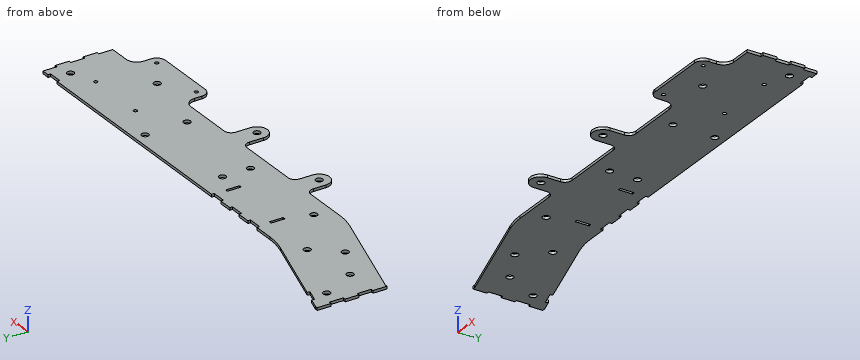
from build123d import *

# Parameters (mm, degrees)
SKETCH2_R                           = 6.35
BASE_DEPTH                          = 4.826
SKETCH3_W                           = 4.826
SKETCH3_H                           = 25.4
CENTER_SUPPORT_VERTICAL_HOLES_DEPTH = 5.826
SKETCH4_W                           = 4.826
SKETCH4_H                           = 25.4
CUT_EXTRUDE2_DEPTH                  = 9.652
SKETCH5_R                           = 3.3528
BOSS_EXTRUDE1_DEPTH                 = 4.826
SKETCH6_R                           = 3.3528
CUT_EXTRUDE3_DEPTH                  = 5.826
SKETCH7_W                           = 25.4
SKETCH7_H                           = 4.826
CUT_EXTRUDE4_DEPTH                  = 4.826


with BuildPart() as part:
    # Sketch2 → base (new body)
    with BuildSketch(Plane.XY):
        with BuildLine():
            Line((-214.699698696, -160.199792202), (-26.873942154, -218.069670807))
            ThreePointArc((-26.873942154, -218.069670807), (-8.387395977, -222.284374422), (10.520610491, -223.699792202))
            Line((10.520610491, -223.699792202), (91.809301303, -223.699792202))
            ThreePointArc((91.809301303, -223.699792202), (100.789557424, -227.419536081), (104.509301303, -236.399792202))
            Line((104.509301303, -236.399792202), (104.509301303, -259.444792203))
            ThreePointArc((104.509301303, -259.444792203), (123.559301303, -278.494792203), (142.609301303, -259.444792203))
            Line((142.609301303, -259.444792203), (142.609301303, -236.399792202))
            ThreePointArc((142.609301303, -236.399792202), (146.329045182, -227.419536081), (155.309301303, -223.699792202))
            Line((155.309301303, -223.699792202), (271.099301303, -223.699792202))
            ThreePointArc((271.099301303, -223.699792202), (280.079557424, -227.419536081), (283.799301303, -236.399792202))
            Line((283.799301303, -236.399792202), (283.799301303, -262.624792203))
            ThreePointArc((283.799301303, -262.624792203), (302.849301303, -281.674792203), (321.899301303, -262.624792203))
            Line((321.899301303, -262.624792203), (321.899301303, -236.399792202))
            ThreePointArc((321.899301303, -236.399792202), (325.619045182, -227.419536081), (334.599301303, -223.699792202))
            Line((334.599301303, -223.699792202), (476.201681216, -223.699792202))
            ThreePointArc((476.201681216, -223.699792202), (482.250146931, -225.232605336), (486.838586238, -229.461042202))
            ThreePointArc((486.838586238, -229.461042202), (518.749301303, -246.744792203), (550.660016368, -229.461042202))
            ThreePointArc((550.660016368, -229.461042202), (555.248455675, -225.232605336), (561.29692139, -223.699792202))
            Line((561.29692139, -223.699792202), (656.774301304, -223.699792202))
            Line((656.774301304, -223.699792202), (656.774301304, -198.299792202))
            Line((656.774301304, -198.299792202), (651.948301304, -198.299792202))
            Line((651.948301304, -198.299792202), (651.948301304, -172.899792202))
            Line((651.948301304, -172.899792202), (656.774301304, -172.899792202))
            Line((656.774301304, -172.899792202), (656.774301304, -147.499792202))
            Line((656.774301304, -147.499792202), (651.948301304, -147.499792202))
            Line((651.948301304, -147.499792202), (651.948301304, -122.099792202))
            Line((651.948301304, -122.099792202), (656.774301304, -122.099792202))
            Line((656.774301304, -122.099792202), (656.774301304, -96.699792202))
            Line((656.774301304, -96.699792202), (174.174301304, -96.699792202))
            Line((174.174301304, -96.699792202), (174.174301304, -101.525792202))
            Line((174.174301304, -101.525792202), (148.774301304, -101.525792202))
            Line((148.774301304, -101.525792202), (148.774301304, -96.699792202))
            Line((148.774301304, -96.699792202), (123.374301304, -96.699792202))
            Line((123.374301304, -96.699792202), (123.374301304, -101.525792202))
            Line((123.374301304, -101.525792202), (97.974301304, -101.525792202))
            Line((97.974301304, -101.525792202), (97.974301304, -96.699792202))
            Line((97.974301304, -96.699792202), (72.574301304, -96.699792202))
            Line((72.574301304, -96.699792202), (72.574301304, -101.525792202))
            Line((72.574301304, -101.525792202), (47.174301304, -101.525792202))
            Line((47.174301304, -101.525792202), (47.174301304, -96.699792202))
            Line((47.174301304, -96.699792202), (10.520610491, -96.699792202))
            ThreePointArc((10.520610491, -96.699792202), (-8.387395977, -95.284374422), (-26.873942154, -91.069670807))
            Line((-26.873942154, -91.069670807), (-169.556754254, -47.108516771))
            Line((-169.556754254, -47.108516771), (-170.977747254, -51.720572158))
            Line((-170.977747254, -51.720572158), (-195.251722975, -44.241661629))
            Line((-195.251722975, -44.241661629), (-193.830729974, -39.629606242))
            Line((-193.830729974, -39.629606242), (-214.699698696, -33.199792202))
            Line((-214.699698696, -33.199792202), (-219.525698696, -33.199792202))
            Line((-219.525698696, -33.199792202), (-219.525698696, -58.599792202))
            Line((-219.525698696, -58.599792202), (-214.699698696, -58.599792202))
            Line((-214.699698696, -58.599792202), (-214.699698696, -83.999792202))
            Line((-214.699698696, -83.999792202), (-219.525698696, -83.999792202))
            Line((-219.525698696, -83.999792202), (-219.525698696, -109.399792202))
            Line((-219.525698696, -109.399792202), (-214.699698696, -109.399792202))
            Line((-214.699698696, -109.399792202), (-214.699698696, -134.799792202))
            Line((-214.699698696, -134.799792202), (-219.525698696, -134.799792202))
            Line((-219.525698696, -134.799792202), (-219.525698696, -160.199792202))
            Line((-219.525698696, -160.199792202), (-214.699698696, -160.199792202))
        make_face()
        with Locations((390.074301304, -191.949792202)):
            Circle(SKETCH2_R, mode=Mode.SUBTRACT)
        with Locations((390.074301304, -115.749792202)):
            Circle(SKETCH2_R, mode=Mode.SUBTRACT)
        with Locations((518.749301303, -221.344792203)):
            Circle(SKETCH2_R, mode=Mode.SUBTRACT)
        with Locations((618.674301304, -128.449792202)):
            Circle(SKETCH2_R, mode=Mode.SUBTRACT)
        with Locations((302.849301303, -262.624792203)):
            Circle(SKETCH2_R, mode=Mode.SUBTRACT)
        with Locations((212.274301304, -191.949792202)):
            Circle(SKETCH2_R, mode=Mode.SUBTRACT)
        with Locations((212.274301304, -141.149792202)):
            Circle(SKETCH2_R, mode=Mode.SUBTRACT)
        with Locations((123.559301303, -259.444792203)):
            Circle(SKETCH2_R, mode=Mode.SUBTRACT)
        with Locations((34.474301304, -191.949792202)):
            Circle(SKETCH2_R, mode=Mode.SUBTRACT)
        with Locations((-92.525698696, -166.549792202)):
            Circle(SKETCH2_R, mode=Mode.SUBTRACT)
        with Locations((-156.850698697, -133.724792203)):
            Circle(SKETCH2_R, mode=Mode.SUBTRACT)
        with Locations((-54.425698696, -122.099792202)):
            Circle(SKETCH2_R, mode=Mode.SUBTRACT)
        with Locations((-187.775698696, -71.299792202)):
            Circle(SKETCH2_R, mode=Mode.SUBTRACT)
    extrude(amount=BASE_DEPTH)

    # Sketch3 → center support vertical holes (cut, through all)
    with BuildSketch(Plane.XY.offset(4.826)):
        with Locations((171.761301304, -134.799792202)):
            Rectangle(SKETCH3_W, SKETCH3_H)
        with Locations((49.587301304, -134.799792202)):
            Rectangle(SKETCH3_W, SKETCH3_H)
    extrude(amount=-CENTER_SUPPORT_VERTICAL_HOLES_DEPTH, mode=Mode.SUBTRACT)

    # Sketch4 → Cut-Extrude2 (cut)
    with BuildSketch(Plane(origin=(656.774301304, 0, 0), x_dir=(0, 0, -1), z_dir=(1, 0, 0))):
        with Locations((-2.413, -109.399792202)):
            Rectangle(SKETCH4_W, SKETCH4_H)
        with Locations((-2.413, -160.199792202)):
            Rectangle(SKETCH4_W, SKETCH4_H)
        with Locations((-2.413, -210.999792202)):
            Rectangle(SKETCH4_W, SKETCH4_H)
    extrude(amount=-CUT_EXTRUDE2_DEPTH, mode=Mode.SUBTRACT)

    # Sketch5 → Boss-Extrude1 (add, through all)
    with BuildSketch(Plane.XY):
        with BuildLine():
            ThreePointArc((447.337201303, -256.561892203), (451.986881152, -267.787212355), (463.212201303, -272.436892203))
            Line((463.212201303, -272.436892203), (574.337201303, -272.436892203))
            ThreePointArc((574.337201303, -272.436892203), (585.562521454, -267.787212355), (590.212201303, -256.561892203))
            Line((590.212201303, -256.561892203), (590.212201303, -242.749792202))
            ThreePointArc((590.212201303, -242.749792202), (595.791817122, -229.279408021), (609.262201303, -223.699792202))
            Line((609.262201303, -223.699792202), (582.274701303, -223.699792202))
            Line((582.274701303, -223.699792202), (582.274701303, -263.705642203))
            ThreePointArc((582.274701303, -263.705642203), (582.042217311, -264.266908211), (581.480951303, -264.499392203))
            Line((581.480951303, -264.499392203), (456.068451303, -264.499392203))
            ThreePointArc((456.068451303, -264.499392203), (455.507185296, -264.266908211), (455.274701303, -263.705642203))
            Line((455.274701303, -263.705642203), (455.274701303, -223.699792202))
            Line((455.274701303, -223.699792202), (428.287201303, -223.699792202))
            ThreePointArc((428.287201303, -223.699792202), (441.757585485, -229.279408021), (447.337201303, -242.749792202))
            Line((447.337201303, -242.749792202), (447.337201303, -256.561892203))
        make_face()
        with BuildLine():
            Line((476.201681216, -223.699792202), (455.274701303, -223.699792202))
            Line((455.274701303, -223.699792202), (455.274701303, -263.705642203))
            ThreePointArc((455.274701303, -263.705642203), (455.507185296, -264.266908211), (456.068451303, -264.499392203))
            Line((456.068451303, -264.499392203), (581.480951303, -264.499392203))
            ThreePointArc((581.480951303, -264.499392203), (582.042217311, -264.266908211), (582.274701303, -263.705642203))
            Line((582.274701303, -263.705642203), (582.274701303, -223.699792202))
            Line((582.274701303, -223.699792202), (561.29692139, -223.699792202))
            ThreePointArc((561.29692139, -223.699792202), (561.2383345, -223.699927338), (561.179748857, -223.700332741))
            ThreePointArc((561.179748857, -223.700332741), (558.402047851, -225.427930059), (555.13360811, -225.295578164))
            ThreePointArc((555.13360811, -225.295578164), (552.64246552, -227.105148928), (550.660016368, -229.461042202))
            ThreePointArc((550.660016368, -229.461042202), (518.749301303, -246.744792203), (486.838586238, -229.461042202))
            ThreePointArc((486.838586238, -229.461042202), (484.864337354, -227.112791145), (482.384586489, -225.306475188))
            ThreePointArc((482.384586489, -225.306475188), (479.131749478, -225.423788448), (476.370155751, -223.700909719))
            ThreePointArc((476.370155751, -223.700909719), (476.285920337, -223.700071584), (476.201681216, -223.699792202))
        make_face()
        with Locations((463.212201303, -256.561892203)):
            Circle(SKETCH5_R, mode=Mode.SUBTRACT)
        with Locations((574.337201303, -256.561892203)):
            Circle(SKETCH5_R, mode=Mode.SUBTRACT)
        with BuildLine():
            ThreePointArc((486.129056336, -220.049392203), (478.617074751, -214.839552456), (476.370155751, -223.700909719))
            ThreePointArc((476.370155751, -223.700909719), (479.47726765, -224.129481142), (482.384586489, -225.306475188))
            ThreePointArc((482.384586489, -225.306475188), (485.097242667, -223.276541717), (486.129056336, -220.049392203))
        make_face()
        with BuildLine():
            ThreePointArc((482.384586489, -225.306475188), (479.47726765, -224.129481142), (476.370155751, -223.700909719))
            ThreePointArc((476.370155751, -223.700909719), (479.131749478, -225.423788448), (482.384586489, -225.306475188))
        make_face()
        with BuildLine():
            ThreePointArc((555.13360811, -225.295578164), (558.402047851, -225.427930059), (561.179748857, -223.700332741))
            ThreePointArc((561.179748857, -223.700332741), (558.056963443, -224.120025409), (555.13360811, -225.295578164))
        make_face()
        with BuildLine():
            ThreePointArc((555.13360811, -225.295578164), (558.056963443, -224.120025409), (561.179748857, -223.700332741))
            ThreePointArc((561.179748857, -223.700332741), (562.192920014, -221.998415637), (562.54554627, -220.049392203))
            ThreePointArc((562.54554627, -220.049392203), (553.769273114, -215.509037195), (555.13360811, -225.295578164))
        make_face()
    extrude(amount=BOSS_EXTRUDE1_DEPTH)

    # Sketch6 → Cut-Extrude3 (cut, through all)
    with BuildSketch(Plane.XY.offset(4.826)):
        with Locations((463.186801303, -145.436892203)):
            Circle(SKETCH6_R)
        with Locations((574.311801303, -145.436892203)):
            Circle(SKETCH6_R)
    extrude(amount=-CUT_EXTRUDE3_DEPTH, mode=Mode.SUBTRACT)

    # Sketch7 → Cut-Extrude4 (cut)
    with BuildSketch(Plane(origin=(0, -96.699792202, 0), x_dir=(1, 0, 0), z_dir=(0, 1, 0))):
        with Locations((620.198301304, -2.413)):
            Rectangle(SKETCH7_W, SKETCH7_H)
    extrude(amount=-CUT_EXTRUDE4_DEPTH, mode=Mode.SUBTRACT)


solid = part.part
The listing builds one solid part. Answer for the finished solid, in the listing's coordinates (mm). Give positions to 0.01 mm unless a question says otherwise; leave off trailing zeros. Order: outer loops, then holes, each group sorted by start corner. A loop starts at its lowest first (then second) coordinate and runs counter-clockwise, first axis right, second up. Notation, with made-up numbers: (-5.75, 28) -> (1.25, 28) arc R21 cw to (1.25, 38) -> close; hole circle Ø3 at (-6.75, 73). An arc over 180 degrees is marked (long way). Put each result on its own line as item: value.
Item 1: A cutting plane is placed at A-A on x = 503.5. Give the vertices of the cut face in (y, z).
Established:
outline: (-272.44, 0) -> (-96.7, 0) -> (-96.7, 4.83) -> (-272.44, 4.83) -> close
Item 2: A cutting plane is placed at C-C on x = -110.5. Give the vertices of the cut face in (y, z).
Established:
outline: (-192.3, 0) -> (-65.3, 0) -> (-65.3, 4.83) -> (-192.3, 4.83) -> close
Item 3: Given P1, Ø11.5, axis at x = 302.85, y = -262.62, coming from the +Z side; P2, Ø1.4, axis at y = -114.5, z = 2, coming from the +X side; P3, Ø2.5, axis at y = -252.5, z = 3, coming from the -X side; P4, Ø1.4, axis at y = -256, z = 2.5, coming from the +X side, each flat-ended and moving along its own axis, determine where each tip first touches the part or whether it passes through.
Established:
P1: passes through
P2: stops at x = 647.12
P3: stops at x = 104.51
P4: stops at x = 590.21
Item 4: Straight lines are drawn through the part: line 1 (Y direction, x = 390, z = 1.85); line 2 (X direction, y = -145, z = 2.3); line 3 (X direction, y = -126, z = 1.15). For each, find the intervals that lie inside material, in ascending order.
Established:
line 1: y = -223.7 to -198.3, -185.6 to -122.1, -109.4 to -96.7
line 2: x = -219.53 to 47.17, 52 to 169.35, 174.17 to 207.22, 217.32 to 459.86, 466.51 to 570.99, 577.64 to 651.95
line 3: x = -214.7 to -59.44, -49.41 to 47.17, 52 to 169.35, 174.17 to 612.82, 624.53 to 651.95
Item 5: A cutting plane is placed at B-B on z = 4.05. Count the separate pieces of the cut face and the enclosed holes in it, plus the area to 3 significant figures.
Established:
separate pieces: 1
enclosed holes: 19
area: 119,000 mm^2
